Can you work these out from the model? Positions are in its coordinate system, mm. Face numbers are marked on the shaded views. A direction names the side the tool comes from. Give positions to 0.01 mm unless a question says otherwise; leave off trailing zeros. Loops run counter-clockwise (first coordinate to the right, second up) from the corner with the lowest first, then second, coordinate; pieces in that order, holes last. Notation, with made-up numbers: (-32.75, 8.25) - (4.25, 8.25) arc R13 ccw to (4.25, 17.25) - close; hole circle Ø8 at (87.5, -32.75). An arc over 180 degrees is marked (long way). Write item = value, one per line.
Autodesk Fusion 360 part; units mm, degrees
sketch "Sketch1" plane through (0, 0, 0) normal (0, 1, 0) x (1, 0, 0)
  line L0 (0, 0) -> (3, 0)
  line L1 (3, 0) -> (3, -16.2727) construction
  line L2 (9.25, -4) -> (-3.25, -4)
  line L3 (-3.25, -4) -> (-3.25, -1.5)
  line L4 (-3.25, -1.5) -> (9.25, -1.5)
  line L5 (9.25, -1.5) -> (9.25, -4)
  line L6 (9.25, -4) -> (-3.25, -1.5) construction
  line L7 (-3.25, -4) -> (9.25, -1.5) construction
  line L8 (0, 0) -> (-2, 2)
  line L9 (-2, 2) -> (-4.45, 2)
  line L10 (-4.45, 2) -> (-4.45, -1.5)
  line L11 (6, 0) -> (3, 0)
  line L12 (6, 0) -> (8, 2)
  line L13 (8, 2) -> (10.45, 2)
  line L14 (10.45, 2) -> (10.45, -1.5)
  line L15 (10.45, -1.5) -> (15.7279, -6.7779)
  arc A0 (-4.45, -10.4359) -> (15.7279, -6.7779) centre (3, 5.95) ccw
  line L16 (-4.45, -1.5) -> (-4.45, -10.4359)
  point P0 (3, -2.75)
  dimension "d3" = 2.5
  dimension "d5" = 12.5
  dimension "d9" = 135
  dimension "d10" = 2
  dimension "d11" = 1.5
  dimension "d12" = 1.2
  dimension "d14" = 3
  dimension "d20" = 18
  dimension "d21" = 45
extrude "Extrude1" add sketch "Sketch1" along normal blind 1.2
sketch "Sketch2" plane through (0, 1.2, 0) normal (0, 1, 0) x (-1, 0, 0)
  line L0 (3.25, 1.5) -> (-9.25, 1.5)
  line L1 (-9.25, 1.5) -> (-9.25, 4)
  line L2 (-9.25, 4) -> (3.25, 4)
  line L3 (3.25, 4) -> (3.25, 1.5)
  line L4 (0, 0) -> (2, -2)
  line L5 (2, -2) -> (4.45, -2)
  line L6 (4.45, -2) -> (4.45, 10.4359)
  line L7 (-15.7279, 6.7779) -> (-10.45, 1.5)
  line L8 (-10.45, 1.5) -> (-10.45, -2)
  line L9 (-10.45, -2) -> (-8, -2)
  line L10 (-8, -2) -> (-6, 0)
  line L11 (-6, 0) -> (0, 0)
  line L12 (-13.5347, 6.2818) -> (-14.8511, 7.5981)
  line L13 (-9.25, 1.9971) -> (-9.25, 1.5)
  line L14 (-9.25, 1.5) -> (3.25, 1.5)
  line L15 (3.25, 1.5) -> (3.25, 1.9971)
  line L16 (-8.4971, -0.8) -> (-6.4971, 1.2) construction
  line L17 (-6.4971, 1.2) -> (0.4971, 1.2) construction
  line L18 (0.4971, 1.2) -> (2.4971, -0.8) construction
  line L19 (2.4971, -0.8) -> (3.25, -0.8)
  line L20 (3.25, -0.8) -> (3.25, 1.9971) construction
  line L21 (-13.5347, 6.2818) -> (-9.25, 1.9971)
  line L22 (-9.25, 1.9971) -> (-9.25, -0.8) construction
  line L23 (-9.25, -0.8) -> (-8.4971, -0.8)
  arc A0 (4.45, 10.4359) -> (-15.7279, 6.7779) centre (-3, -5.95) ccw
  arc A1 (3.9533, 9.3435) -> (-14.8794, 5.9294) centre (-3, -5.95) ccw
  line L24 (3.25, 1.5) -> (3.25, 10.9301)
  dimension "d22" = 1.2
  dimension "d24" = -1.2
extrude "Extrude2" add sketch "Sketch2" along normal blind 12.5 contours L0 L1 L3 L4 L5 L6 L7 L8 L9 L10 L11 L12 L13 L14 L15 L21 A0 A1 L24 | L7 L12 A0 A1
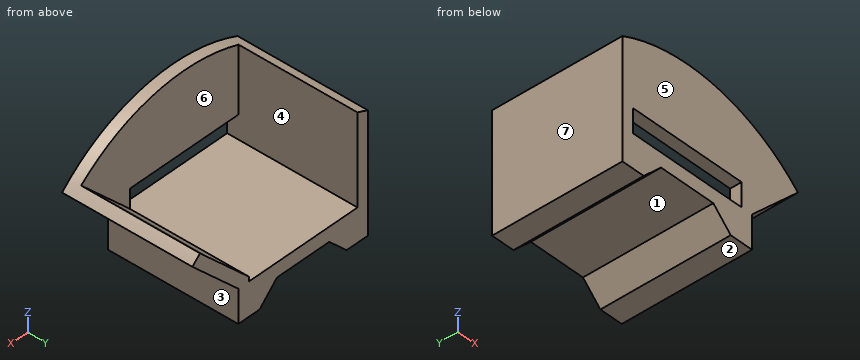
Q1. For pin 1 (5 mm diameter, centred on x = 4, z = 4.5, fed in from +Y); pin 2 (4 mm diameter, centred on y = 12, z = 9.5, fed in from +X); pin 3 (0.6 mm diameter, centred on x = 6, y = 0.5, fed in from -Z), each with a flat end and sliding along its axis, tell me the tip position at first contact or that it passes through.
Output:
pin_1 = 1.2
pin_2 = 14.96
pin_3 = -0.3
Q2. We'd pull the mould along X, two halves only. Please class the marked faces 4, 5, 6 and 7: released by +X, released by -X, zero draft, split by the parting line, or undercut.
Output:
face_4 = undercut
face_5 = zero draft
face_6 = undercut
face_7 = released by -X
Q3. Imagine slicing it at A-A, the plane x = -2.75. Write out the boundary of the cut face in (y, z).
Output:
outline = (0, -2) - (13.7, -2) - (13.7, 1.5) - (0, 1.5) - close; (0, 4) - (1.2, 4) - (1.2, 11.11) - (0, 11.11) - close
Q4. Imagine slicing it at B-B, the plane z = 3.25. Write out the boundary of the cut face in (x, y), then the cut area to 3 significant figures.
Output:
outline = (-4.45, 0) - (-3.25, 0) - (-3.25, 13.7) - (-4.45, 13.7) - close; (9.25, 0) - (12.2, 0) - (12.2, 13.7) - (10.5, 13.7) - (10.5, 1.2) - (9.25, 1.2) - close
area = 41.2 mm2
Q5. Imagine slicing it at D-D, the plane x = 2.75. Write out the boundary of the cut face in (y, z).
Output:
outline = (0, 0) - (13.7, 0) - (13.7, 1.5) - (0, 1.5) - close; (0, 4) - (1.2, 4) - (1.2, 12.05) - (0, 12.05) - close
Q6. Which directions (+Z, -Z, +X, -X, +Y, -Y) give clear straight access to the entire face, cutting with the end or side of a thin tool? Please do the marked faces 1, 2 and 3.
Output:
face_1 = -Z, +Y, -Y
face_2 = -Z, +X, -X, +Y, -Y
face_3 = -Z, +X, +Y, -Y
Q7. Imagine slicing it at C-C, the plane y = 2.75. Write out the boundary of the cut face in (x, z).
Output:
outline = (-4.45, -2) - (-2, -2) - (0, 0) - (6, 0) - (8, -2) - (10.45, -2) - (10.45, 1.5) - (15.73, 6.78) arc R18 ccw to (14.85, 7.6) - (13.53, 6.28) - (9.25, 2) - (9.25, 1.5) - (-3.25, 1.5) - (-3.25, 10.93) arc R18 ccw to (-4.45, 10.44) - close
Q8. I need wall thicknesses on L1, parallel to Z at x = 5.25, y = 4; L2, parallel to X at y = 2.25, z = 8; L3, parallel to X at y = 4.5, z = 6.75. Which ranges of each line are inside material? Lowest first, please.
Output:
L1 = 0 to 1.5
L2 = -4.45 to -3.25
L3 = -4.45 to -3.25, 14 to 15.7
